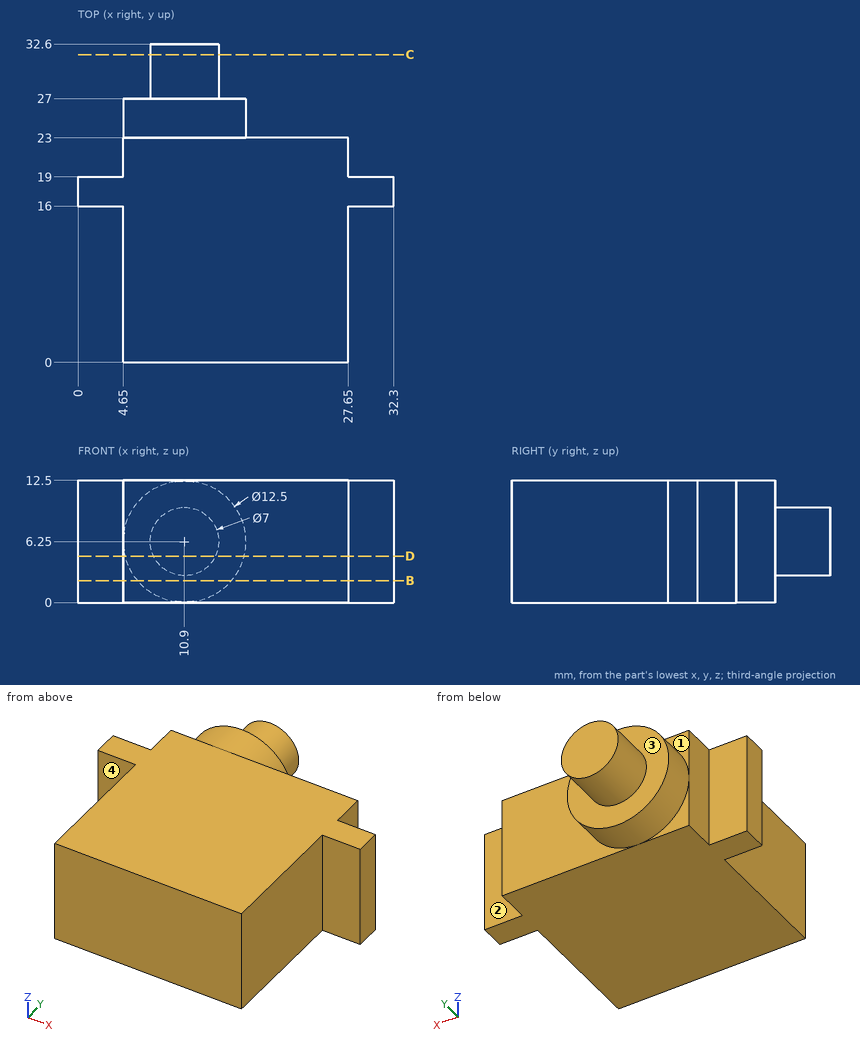
Source: three-view drawing plus pictorial views. Frame: mm from the lowest corner of the part. A direction names the side the tool comes from. Coordinates: 2 decimals unless noted, no trailing zeros. Loops run counter-clockwise (first coordinate to the right, second up) from the corner with the lowest first, then second, coordinate; pieces in that order, holes last. Notation, with made-up numbers: (48, -7) - (72, -7) arc R22 cw to (72, 20) - close; hole circle Ø9 at (-35, 44.5). An arc over 180 degrees is marked (long way). One line per question, with ' | ' between items.
1) Section B-B, the plane z = 2.25. Return loops of the section in (x, y), then the cut area to 3 significant figures.
Report:
outline: (0, 16) - (4.65, 16) - (4.65, 0) - (27.65, 0) - (27.65, 16) - (32.3, 16) - (32.3, 19) - (27.65, 19) - (27.65, 23) - (15.7, 23) - (15.7, 27) - (6.1, 27) - (6.1, 23) - (4.65, 23) - (4.65, 19) - (0, 19) - close | area: 595 mm²
2) Line query: line 1 along X through (y, z) = (9, 7); line 2 along Y through (x, z) = (2.5, 2.75); line 3 along Y through (x, z) = (9.5, 10.75). Output: solid intervals per line, ascending.
Report:
line 1: x = 4.65 to 27.65 | line 2: y = 16 to 19 | line 3: y = 0 to 27
3) Section C-C, the plane y = 31.5. Return loops of the section in (x, z), then the cut area to 3 significant figures.
Report:
outline: circle Ø7 at (10.9, 6.25) | area: 38.5 mm²
4) Set-up query: the marked faces 1, 2, 3 and 4. Return all of +Z, -Z, +X, -X, +Y, -Y with unobstructed straight access to the full face (end or side cutting, diameter ignored); none if empty.
Report:
face 1: +Z, -X, +Y | face 2: +Z, -Z, +X, +Y | face 3: +Y | face 4: +Z, -Z, -X, -Y
5) Section D-D, the plane z = 4.75. Return loops of the section in (x, y).
Report:
outline: (0, 16) - (4.65, 16) - (4.65, 0) - (27.65, 0) - (27.65, 16) - (32.3, 16) - (32.3, 19) - (27.65, 19) - (27.65, 23) - (16.97, 23) - (16.97, 27) - (14.06, 27) - (14.06, 32.6) - (7.74, 32.6) - (7.74, 27) - (4.83, 27) - (4.83, 23) - (4.65, 23) - (4.65, 19) - (0, 19) - close
6) First-contact query: P1, Ø2, axis at y = 21, z = 6, coming from the -X side; P2, Ø4.5, axis at y = 21.5, z = 5.5, coming from the +X side; P3, Ø1.4, axis at x = 31, z = 9.5, coming from the -Y side. Flat tips, straight axial feed; report the tip coordinate or a pass-through.
Report:
P1: stops at x = 4.65 | P2: stops at x = 27.65 | P3: stops at y = 16
